from build123d import *

# Parameters (mm, degrees)
BOSS_EXTRUDE1_DEPTH = 4
CUT_EXTRUDE1_REACH  = 67.872
SKETCH2_R           = 1.1
SKETCH2_W           = 12
SKETCH2_H           = 23
FILLET1_R           = 2
FILLET2_R           = 1
FILLET3_R           = 1
SKETCH3_W           = 3.666320095
SKETCH3_H           = 10
SKETCH3_W_2         = 4
BOSS_EXTRUDE2_DEPTH = 12
SKETCH4_W           = 19.666320095
SKETCH4_H           = 10
BOSS_EXTRUDE3_DEPTH = 2
SKETCH5_R           = 3.4
BOSS_EXTRUDE4_DEPTH = 2


with BuildPart() as part:
    # Sketch1 → Boss-Extrude1 (new body)
    with BuildSketch(Plane.XY):
        with BuildLine():
            Line((10.219576084, 1.434709353), (10.219576084, -58.565290647))
            Line((10.219576084, -58.565290647), (14.921299434, -58.565290647))
            Line((14.921299434, -58.565290647), (14.921299434, -58.307205095))
            add(Edge.make_bspline(
                [(29.885896179, -28.969975988), (15.603913992, -34.528623974), (14.921299434, -58.307205095)],
                knots=[0, 0, 0, 1, 1, 1], degree=2))
            Line((29.885896179, -28.969975988), (29.885896179, 1.434709353))
            ThreePointArc((29.885896179, 1.434709353), (20.052736131, 11.2678694), (10.219576084, 1.434709353))
        make_face()
    extrude(amount=BOSS_EXTRUDE1_DEPTH)

    # Sketch2 → Cut-Extrude1 (cut, up to next)
    with BuildSketch(Plane.XY.offset(4), mode=Mode.PRIVATE) as cut_extrude1_sk1:
        with Locations((20.219576084, 4.084709353)):
            Circle(SKETCH2_R)
    cut_extrude1_tool1 = extrude(cut_extrude1_sk1.sketch, amount=-CUT_EXTRUDE1_REACH, mode=Mode.PRIVATE) & part.part
    # Sketch2 → Cut-Extrude1 (cut, up to next)
    with BuildSketch(Plane.XY.offset(4), mode=Mode.PRIVATE) as cut_extrude1_sk2:
        with Locations((20.219576084, -24.215290647)):
            Circle(SKETCH2_R)
    cut_extrude1_tool2 = extrude(cut_extrude1_sk2.sketch, amount=-CUT_EXTRUDE1_REACH, mode=Mode.PRIVATE) & part.part
    # Sketch2 → Cut-Extrude1 (cut, up to next)
    with BuildSketch(Plane.XY.offset(4), mode=Mode.PRIVATE) as cut_extrude1_sk3:
        with Locations((20.219576084, -10.065290647)):
            Rectangle(SKETCH2_W, SKETCH2_H)
    cut_extrude1_tool3 = extrude(cut_extrude1_sk3.sketch, amount=-CUT_EXTRUDE1_REACH, mode=Mode.PRIVATE) & part.part
    add(cut_extrude1_tool1.solids().sort_by_distance((20.219576, 4.084709, 4))[0], mode=Mode.SUBTRACT)
    add(cut_extrude1_tool2.solids().sort_by_distance((20.219576, -24.215291, 4))[0], mode=Mode.SUBTRACT)
    add(cut_extrude1_tool3.solids().sort_by_distance((20.219576, -10.065291, 4))[0], mode=Mode.SUBTRACT)

    # Fillet1
    fillet1_edges = [part.edges().sort_by_distance(p)[0] for p in [
        (29.885896179, -28.969975988, 2),
    ]]
    fillet(fillet1_edges, radius=FILLET1_R)

    # Fillet2
    fillet2_edges = [part.edges().sort_by_distance(p)[0] for p in [
        (14.921299434, -58.565290647, 2),
    ]]
    fillet(fillet2_edges, radius=FILLET2_R)

    # Fillet3
    fillet3_edges = [part.edges().sort_by_distance(p)[0] for p in [
        (10.219576084, -58.565290647, 2),
    ]]
    fillet(fillet3_edges, radius=FILLET3_R)

    # Sketch3 → Boss-Extrude2 (add)
    with BuildSketch(Plane(origin=(0, 0, 0), x_dir=(-1, 0, 0), z_dir=(0, 0, -1))):
        with Locations((-28.052736132, -4.865290647)):
            Rectangle(SKETCH3_W, SKETCH3_H)
        with Locations((-12.219576084, -4.865290647)):
            Rectangle(SKETCH3_W_2, SKETCH3_H)
    extrude(amount=BOSS_EXTRUDE2_DEPTH)

    # Sketch4 → Boss-Extrude3 (add)
    with BuildSketch(Plane(origin=(0, 0, -12), x_dir=(-1, 0, 0), z_dir=(0, 0, -1))):
        with Locations((-20.052736132, -4.865290647)):
            Rectangle(SKETCH4_W, SKETCH4_H)
    extrude(amount=BOSS_EXTRUDE3_DEPTH)

    # Sketch5 → Boss-Extrude4 (add)
    with BuildSketch(Plane(origin=(0, 0, -14), x_dir=(-1, 0, 0), z_dir=(0, 0, -1))):
        with Locations((-20.285896179, -4.665290647)):
            Circle(SKETCH5_R)
    extrude(amount=BOSS_EXTRUDE4_DEPTH)


solid = part.part
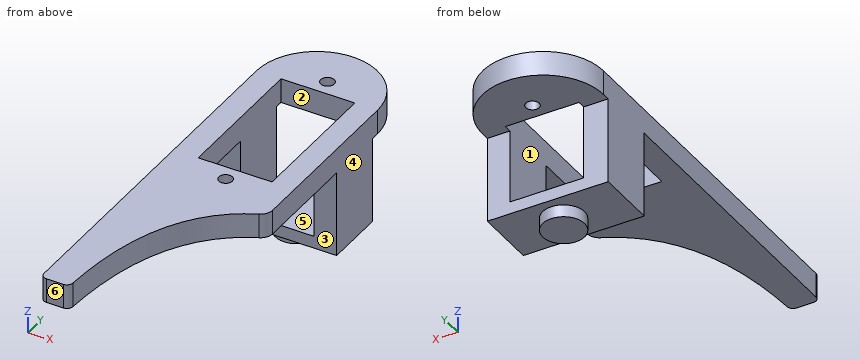
Geometry: final body of the model. Coordinates: model frame, mm. Face numbers are marked on the shaded views. A direction names the side the tool comes from. Coordinates: 2 decimals unless noted, no trailing zeros. Loops run counter-clockwise (first coordinate to the right, second up) from the corner with the lowest first, then second, coordinate; pieces in that order, holes last. Notation, with made-up numbers: M 84,39 L 104,39 A19 ccw 104,72 Z; hole C 43,83.5 d5. An arc over 180 degrees is marked long. One line per item, written item: value. Start each with the question number.
1) Cut plane B-B (x = 12). Return loops of the section in (y, z), then the cut area to 3 significant figures.
2) Draft query along X for the marked faces 4, 5 and 6. Return one class per face: released by +X, released by -X, zero draft, split by the parting line, or undercut.
3) Pin query (flat end, axial travel): P1, Ø5, axis at x = 17.5, y = -3.5, coming from the +Z side; P2, Ø1.5, axis at x = 14.5, y = -13, coming from the -Z side; P3, Ø10, axis at x = 14.5, z = 2, coming from the +Y side. Return the tip coordinate at first contact, or that it passes through.
4) Cut plane C-C (y = -5.5). Return loops of the section in (x, z), then the cut area to 3 significant figures.
5) Material intervals for L1, parallel to Z at x = 12.5, y = -44; L2, parallel to X at y = -1.5, z = 1.5; L3, parallel to Y at x = 12.5, z = -3.75, sorted ascending. Write a range as from..to.
6) Cut plane A-A (z = -2.5). Return loops of the section in (x, y).
7) Cut plane D-D (x = 23). Count the separate pieces of the cut face and the enclosed holes in it, then the cut area to 3 significant figures.
8) Reachability of the marked faces 1, 2 and 3 from +Z, -Z, +X, -X, +Y, -Y: full face, straight path, thin tool, end or side. Return the list, or none.
Evaluation:
1. outline: M -58.57,0 L -9.87,0 L -9.87,-14 L 0.13,-14 L 0.13,0 L 7.08,0 L 7.08,4 L -58.57,4 Z
1. area: 403 mm^2
2. face 4: released by +X
2. face 5: undercut
2. face 6: zero draft
3. P1: z = -12
3. P2: z = 0
3. P3: y = 11.25
4. outline: M 10.22,-14 L 16.99,-14 L 16.99,-16 L 23.58,-16 L 23.58,-14 L 29.89,-14 L 29.89,4 L 26.22,4 L 26.22,-12 L 14.22,-12 L 14.22,4 L 10.22,4 Z
4. area: 175 mm^2
5. L1: 0..4
5. L2: 10.22..14.22, 26.22..29.89
5. L3: -9.87..0.13
6. outline: M 10.22,-9.87 L 14.22,-9.87 L 14.22,0.13 L 10.22,0.13 Z; M 26.22,-9.87 L 29.89,-9.87 L 29.89,0.13 L 26.22,0.13 Z
7. separate pieces: 3
7. enclosed holes: 0
7. area: 113 mm^2
8. face 1: +Z
8. face 2: +Z, -Z
8. face 3: -Z, +X, -X, -Y
